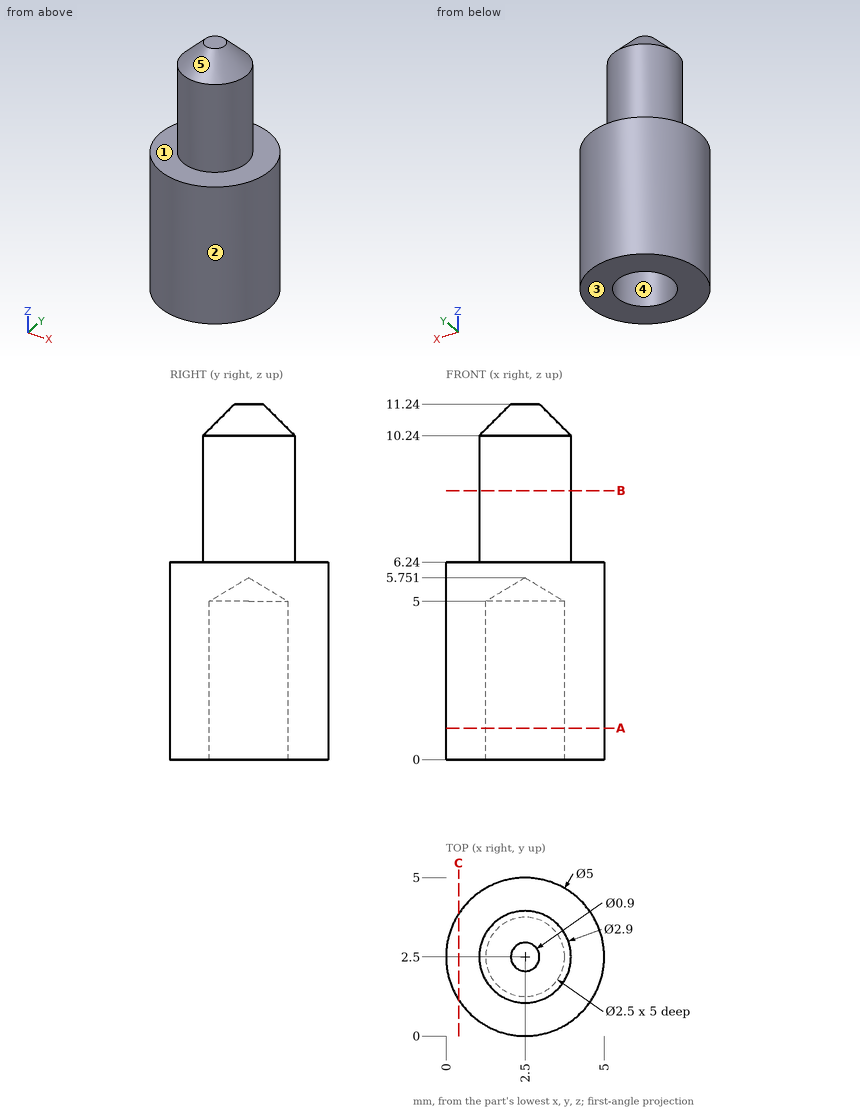
Answer from the drawing. Dimensions are ordinates in mm from the lowest x, y and z of the part. A direction names the side the tool comes from. Coordinates: 2 decimals unless noted, no trailing zeros. Order: outer loops, then holes, each group sorted by start corner. A loop starts at its lowest first (then second) coordinate and runs counter-clockwise, first axis right, second up. Notation, with made-up numbers: (-35.75, 0) - (-27.75, 0) arc R30 cw to (-27.75, 26) - close; hole circle Ø2 at (-6.5, -8.5). An arc over 180 degrees is marked (long way). Put each result on its own line as item: value. Start each with the question number.
1) Find section B-B (z = 8.5). Give the vertices of the cut face in (x, y).
2) For a pull along X with two mould halves and no side action, classify the marked faces 3, 4 and 5 as released by +X, released by -X, zero draft, split by the parting line, or undercut.
3) Find the intervals of material crossed by line 1 (Y direction, x = 2.5, z = 1.3); line 2 (Z direction, x = 1.8, y = 1.15); line 3 (X direction, y = 1.75, z = 3.25) (1 decimal), in increasing order. Write a range as from..to.
4) Find section A-A (z = 1). Give the vertices of the cut face in (x, y).
5) Find section C-C (x = 0.4). Give the vertices of the cut face in (y, z).
6) Flat-ended cylindrical pins translate along their axes: pin 1 (1.5 mm diameter, centred on x = 2, z = 8.5, fed in from +Y); pin 2 (3 mm diameter, centred on x = 0.5, y = 4, fed in from +Z); pin 3 (1 mm diameter, centred on x = 3.5, y = 2, fed in from +Z). Find the tip coordinate at first contact, or state that the pin passes through.
7) For the marked faces 1 and 2, determine the directions among +Z, -Z, +X, -X, +Y, -Y from which every point of the face is accessible in a straight line to the end or side of a thin tool.
Results list:
1. outline: circle Ø2.9 at (2.5, 2.5)
2. face 3: zero draft
2. face 4: undercut
2. face 5: split by the parting line
3. line 1: y = 0..1.25, 3.75..5
3. line 2: z = 0..6.24
3. line 3: x = 0.1..1.5, 3.5..4.9
4. outline: circle Ø5 at (2.5, 2.5); hole circle Ø2.5 at (2.5, 2.5)
5. outline: (1.14, 0) - (3.86, 0) - (3.86, 6.24) - (1.14, 6.24) - close
6. pin 1: stops at y = 3.95
6. pin 2: stops at z = 10.69
6. pin 3: stops at z = 11.07
7. face 1: +Z
7. face 2: +Z, -Z
